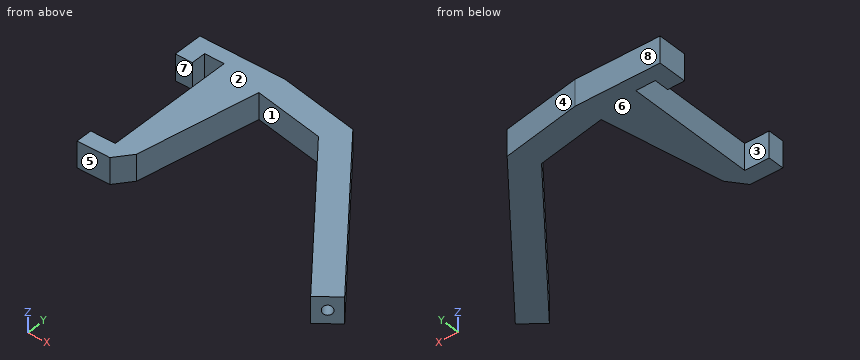
```python
from build123d import *

# Parameters (mm, degrees)
F1_DEPTH = 8
F3_D     = 3
F3_DEPTH = 6
F3_TIP   = 0.9012909285


with BuildPart() as f1:
    # F0 (on Top) → F1 (new body)
    with BuildSketch(Plane.XY):
        Polygon((-35.0272064194, 47.1324694753), (-35.0272064194, 51.6324694753), (-29.0272064194, 51.6324694753), (-29.0272064194, 11.6324694753), (-36.5272064194, 11.6324694753), (-36.5272064194, 6.6324694753), (-26.5272064194, 6.6324694753), (-22.5272064194, 11.6324694753), (-15.6577646998, 48.2694919798), (5.9506252409, 44.2179188659), (43.934325687, -4.2605536739), (50.2315890367, 0.6734583148), (10.388348254, 51.525256099), (-14.1834564194, 56.1324694753), (-40.2272064194, 56.1324694753), (-40.2272064194, 47.1324694753), align=None)
    extrude(amount=F1_DEPTH)

    # F3
    with Locations(Plane(origin=(18.7802618476, -23.969186719, 0), x_dir=(0.7871579187, 0.6167514986, 0), z_dir=(0.6167514986, -0.7871579187, 0))):
        with Locations((35.9555495046, 4)):
            Hole(F3_D / 2, depth=F3_DEPTH)
            with Locations((0, 0, -(F3_DEPTH + F3_TIP / 2))):  # 118° drill point
                Cone(0, F3_D / 2, F3_TIP, mode=Mode.SUBTRACT)


solid = f1.part
```
For this review, take the finished solid that the model builds, in its own axes (mm). Face numbers are marked on the shaded views. A direction names the side the tool comes from. Round coordinates to 2 decimals unless told otherwise and drop trailing zeros. Order: outer loops, then holes, each group sorted by start corner. A loop starts at its lowest first (then second) coordinate and runs counter-clockwise, first axis right, second up. Notation, with made-up numbers: (-36, 70) -> (-16, 70) arc R21 cw to (-16, 75) -> close; hole circle Ø9 at (36.5, 38.5). An arc over 180 degrees is marked (long way). Use a Markdown table: item, result.
Item 1: Take a section at B-B (y = 29). State the section outline as (x, z) points.
Resolved:
| item | result |
|---|---|
| outline | (-29.03, 0) -> (-19.27, 0) -> (-19.27, 8) -> (-29.03, 8) -> close; (17.87, 0) -> (28.04, 0) -> (28.04, 8) -> (17.87, 8) -> close |
Item 2: Draft analysis for pull direction Y (two halves, no side actions). For the marked faces 6, 7 and 8, state which applies: +Y half, -Y half, draft (parallel to the pull), parting line (faces both ways), or undercut.
Resolved:
| item | result |
|---|---|
| face 6 | draft |
| face 7 | undercut |
| face 8 | +Y half |
Item 3: Machinability: for the marked faces 1, 2, 3, 4 and 5, which of the approach directions +Z, -Z, +X, -X, +Y, -Y give a long, thin tool a straight path to every point of the face, cutting with its end or side? Answer none if there is none.
Resolved:
| item | result |
|---|---|
| face 1 | +Z, -Z, -Y |
| face 2 | +Z, +X, -X, +Y, -Y |
| face 3 | +Z, -Z, -X |
| face 4 | +Z, -Z, +X, +Y |
| face 5 | +Z, -Z, -X, -Y |
Item 4: Take a section at D-D (x = 41). State the section outline as (y, z) points, plus the area to 3 significant figures.
Resolved:
| item | result |
|---|---|
| outline | (-0.52, 0) -> (12.46, 0) -> (12.46, 8) -> (-0.52, 8) -> close |
| area | 104 mm² |
Item 5: For pin 1 (1 mm diameter, centred on x = -7, z = 3.5, fed in from +Y); pin 2 (1.8 mm diameter, centred on x = -31, z = 5.5, fed in from -Y); pin 3 (1 mm diameter, centred on x = -16, y = 43, fed in from -Z); pin 4 (2.5 mm diameter, centred on y = 38.5, z = 4.5, fed in from -X), all flat-tipped, find the tip position at first contact; note any pin that passes through.
Resolved:
| item | result |
|---|---|
| pin 1 | stops at y = 54.88 |
| pin 2 | stops at y = 6.63 |
| pin 3 | passes through |
| pin 4 | stops at x = -29.03 |
Item 6: Take a section at C-C (x = -19). State the section outline as (y, z) points, plus the area to 3 significant figures.
Resolved:
| item | result |
|---|---|
| outline | (30.44, 0) -> (56.13, 0) -> (56.13, 8) -> (30.44, 8) -> close |
| area | 206 mm² |
Item 7: Take a section at A-A (x = -32.5). State the section outline as (y, z) points.
Resolved:
| item | result |
|---|---|
| outline | (6.63, 0) -> (11.63, 0) -> (11.63, 8) -> (6.63, 8) -> close; (51.63, 0) -> (56.13, 0) -> (56.13, 8) -> (51.63, 8) -> close |
Item 8: For line 1 along Y through (x, z) = (-27, 7.25); line 2 along X through (y, z) = (28, 1.5); line 3 along X through (y, z) = (7, 2.25), list the stretches that pass through material, from the lowest coordinate up. Write a range as [from, to].
Resolved:
| item | result |
|---|---|
| line 1 | y = [6.63, 56.13] |
| line 2 | x = [-29.03, -19.46], [18.66, 28.82] |
| line 3 | x = [-36.53, -26.23], [35.11, 45.27] |
